Could you check a few things on this model? Use its own coordinates, in mm. Face numbers are marked on the shaded views. A direction names the side the tool comes from. Coordinates: 2 decimals unless noted, no trailing zeros. Order: outer loops, then holes, each group sorted by start corner. A loop starts at its lowest first (then second) coordinate and runs counter-clockwise, first axis right, second up. Notation, with made-up numbers: (80.5, 55) -> (138.5, 55) arc R22 ccw to (138.5, 68) -> close; hole circle Ø2 at (-37, -23). An arc over 180 degrees is marked (long way). Use a Markdown table: item, result. Add a question column.
1) If I drill on L1, parallel to Y at x = -32, z = 26.5; L2, parallel to X at y = -14, z = 17; L3, parallel to Z at x = -3, y = -7, over which ranges is the centre line in solid material (lowest first)? Write a range as [from, to].
2) If we section it at C-C (x = 8): Write out the boundary of the cut face in (y, z).
3) If we section it at B-B (y = 3): Write out the boundary of the cut face in (x, z), plus the area to 3 significant figures.
4) Which directions (+Z, -Z, +X, -X, +Y, -Y) give clear straight access to the entire face, cutting with the end or side of a thin tool? Please do the marked faces 4 and 5.
5) If we section it at A-A (z = 25): Write out the boundary of the cut face in (x, y), plus the area to 3 significant figures.
6) Thinking about a two-plate mould opening in X: for the marked faces 1, 2 and 3, which applies, +X half, -X half, draft (parallel to the pull), parting line (faces both ways), or undercut?
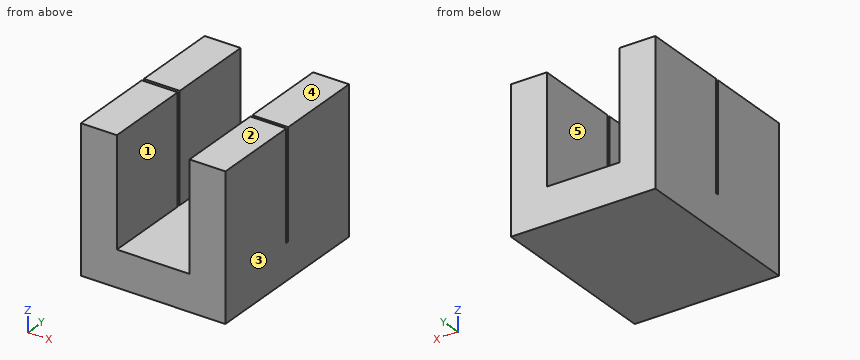
```python
from build123d import *

# Parameters (mm, degrees)
F1_DEPTH = 50
F2_DEPTH = 0.8


with BuildPart() as f1:
    # F0 (on Front) → F1 (new body, symmetric)
    with BuildSketch(Plane.XZ):
        Polygon((-20.2, -20), (-20.2, 20), (-20.2, 40), (-40.2, 40), (-40.2, -20), align=None)
        Polygon((40.2, -20), (20.2, -20), (-20.2, -20), (-40.2, -20), (-40.2, -40), (40.2, -40), align=None)
        Polygon((20.2, 40), (20.2, 20), (20.2, -20), (40.2, -20), (40.2, 40), align=None)
    extrude(amount=F1_DEPTH, both=True)

    # F0 (on Front) → F2 (cut, symmetric)
    with BuildSketch(Plane.XZ):
        Polygon((-20.2, -20), (-20.2, 20), (-20.2, 40), (-40.2, 40), (-40.2, -20), align=None)
        Polygon((20.2, 40), (20.2, 20), (20.2, -20), (40.2, -20), (40.2, 40), align=None)
    extrude(amount=F2_DEPTH, both=True, mode=Mode.SUBTRACT)


solid = f1.part
```
Answer sheet:
| question | item | result |
|---|---|---|
| 1 | L1 | [-50, -0.8], [0.8, 50] |
| 1 | L2 | [-40.2, -20.2], [20.2, 40.2] |
| 1 | L3 | [-40, -20] |
| 2 | outline | (-50, -40) -> (50, -40) -> (50, -20) -> (-50, -20) -> close |
| 3 | outline | (-40.2, -40) -> (40.2, -40) -> (40.2, 40) -> (20.2, 40) -> (20.2, -20) -> (-20.2, -20) -> (-20.2, 40) -> (-40.2, 40) -> close |
| 3 | area | 4,010 mm2 |
| 4 | face 4 | +Z, +X, -X, +Y, -Y |
| 4 | face 5 | +Z, +Y, -Y |
| 5 | outline | (-40.2, -50) -> (-20.2, -50) -> (-20.2, -0.8) -> (-40.2, -0.8) -> close; (-40.2, 0.8) -> (-20.2, 0.8) -> (-20.2, 50) -> (-40.2, 50) -> close; (20.2, -50) -> (40.2, -50) -> (40.2, -0.8) -> (20.2, -0.8) -> close; (20.2, 0.8) -> (40.2, 0.8) -> (40.2, 50) -> (20.2, 50) -> close |
| 5 | area | 3,940 mm2 |
| 6 | face 1 | undercut |
| 6 | face 2 | draft |
| 6 | face 3 | +X half |
